```python
from build123d import *

# Parameters (mm, degrees)
F0_W     = 17.30713
F0_H     = 5.958192
F1_DEPTH = 13.335
F2_DEPTH = 13.335
F3_R     = 5.08
F4_R     = 1.905
F5_DEPTH = 19.05
F6_R     = 1.905


with BuildPart() as f1:
    # F0 (on Front) → F1 (new body)
    with BuildSketch(Plane.XZ):
        Rectangle(F0_W, F0_H)
    extrude(amount=F1_DEPTH)

    # F0 (on Front) → F2 (join)
    with BuildSketch(Plane.XZ):
        Rectangle(F0_W, F0_H)
    extrude(amount=-F2_DEPTH)

    # F3
    f3_edges = [f1.edges().sort_by_distance(p)[0] for p in [
        (8.653565, 0, 2.979096),
        (0, 13.335, 2.979096),
        (-8.653565, 0, 2.979096),
        (0, -13.335, 2.979096),
    ]]
    fillet(f3_edges, radius=F3_R)

    # F4 (on face) → F5 (join)
    with BuildSketch(Plane(origin=(0, 0, -2.979096), x_dir=(1, 0, 0), z_dir=(0, 0, -1))):
        with Locations((0, 10.16)):
            Circle(F4_R)
        with Locations((0, -9.525)):
            Circle(F4_R)
    extrude(amount=F5_DEPTH)

    # F6
    f6_edges = [f1.edges().sort_by_distance(p)[0] for p in [
        (-1.905, -10.16, -22.029096),
        (-1.905, 9.525, -22.029096),
    ]]
    fillet(f6_edges, radius=F6_R)


solid = f1.part
```
Geometry: final body of the model. Coordinates: model frame, mm. A direction names the side the tool comes from. Round coordinates to 2 decimals unless told otherwise and drop trailing zeros. Loops run counter-clockwise (first coordinate to the right, second up) from the corner with the lowest first, then second, coordinate; pieces in that order, holes last. Notation, with made-up numbers: (70.25, 58) -> (98.25, 58) arc R24 cw to (98.25, 68) -> close; hole circle Ø5 at (-21, 89.25). An arc over 180 degrees is marked (long way). Write each question's results on one line, items separated by ' | '.
Item 1: Cut plane B-B on x = 0. Return the cut outline in (y, z) (3 decimals), and give its area (3 significant figures).
Answers below:
outline: (-13.335, -2.979) -> (-12.065, -2.979) -> (-12.065, -20.124) arc R1.905 ccw to (-8.255, -20.124) -> (-8.255, -2.979) -> (7.62, -2.979) -> (7.62, -20.124) arc R1.905 ccw to (11.43, -20.124) -> (11.43, -2.979) -> (13.335, -2.979) -> (13.335, -2.101) arc R5.08 ccw to (8.255, 2.979) -> (-8.255, 2.979) arc R5.08 ccw to (-13.335, -2.101) -> close | area: 290 mm²
Item 2: Pull-direction query (Y, two-part tool) for faces 1 (the face through (0, 0, 2.979)), 2 (the face through (-0.25, -12.05, -11.43)), 3 (the face through (-0.1, -13.335, -2.5)); classes: pulls with the +Y half, pulls with the -Y half, needs draft (parallel to the pull), parting line crosses it, or undercut.
Answers below:
face 1: needs draft | face 2: undercut | face 3: pulls with the -Y half
Item 3: Cut plane C-C on z = -10. Return the cut outline in (x, y) (3 decimals).
Answers below:
outline: circle Ø3.81 at (0, -10.16); circle Ø3.81 at (0, 9.525)
Item 4: Pin query (flat end, axial travel): pin 1 Ø2 at (y, z) = (7, -16.5) entering from +X; pin 2 Ø8 at (x, z) = (0, -16.5) entering from -Y (3 decimals); pin 3 Ø2 at (x, z) = (-2.5, -15) entering from +Y. Return the tip coordinate at first contact, or that it passes through.
Answers below:
pin 1: stops at x = 1.14 | pin 2: stops at y = -12.065 | pin 3: stops at y = 10.7
Item 5: Set-up query: faces 4 (the face through (-0.413, 11.385, -11.432)), 5 (the face through (-0.1, 13.335, -2.5)). Return all of +Z, -Z, +X, -X, +Y, -Y with unobstructed straight access to the full face (end or side cutting, diameter ignored); none if empty.
Answers below:
face 4: -Z | face 5: +Z, -Z, +X, -X, +Y
Item 6: Line query: probe 1 along Z at (x, y) = (-3, 0.5); probe 2 along Y at (x, z) = (1.5, -8.25); probe 3 along Y at (x, z) = (-0.25, -8.75). Output: solid intervals per line, ascending. Write a range as [from, to].
Answers below:
probe 1: z = [-2.98, 2.98] | probe 2: y = [-11.33, -8.99], [8.35, 10.7] | probe 3: y = [-12.05, -8.27], [7.64, 11.41]
Item 7: Cut plane D-D on y = -10.16. Return the cut outline in (x, z) (3 decimals), and give its area (3 significant figures).
Answers below:
outline: (-8.654, -2.979) -> (-1.905, -2.979) -> (-1.905, -20.124) arc R1.905 ccw to (1.905, -20.124) -> (1.905, -2.979) -> (8.654, -2.979) -> (8.654, -2.101) arc R5.08 ccw to (5.479, 2.608) -> (-5.479, 2.608) arc R5.08 ccw to (-8.654, -2.101) -> close | area: 159 mm²
Item 8: Cut plane A-A on y = 2.25. Return the cut outline in (x, z), and give its area (3 significant figures).
Answers below:
outline: (-8.65, -2.98) -> (8.65, -2.98) -> (8.65, -2.1) arc R5.08 ccw to (3.57, 2.98) -> (-3.57, 2.98) arc R5.08 ccw to (-8.65, -2.1) -> close | area: 92.0 mm²
